Answer from the drawing. Dimensions are ordinates in mm from the lowest x, y and z of the part. A direction names the side the tool comes from. Round coordinates to 2 decimals unless told otherwise and drop trailing zeros. Loops run counter-clockwise (first coordinate to the right, second up) from the corner with the lowest first, then second, coordinate; pieces in that order, holes last.
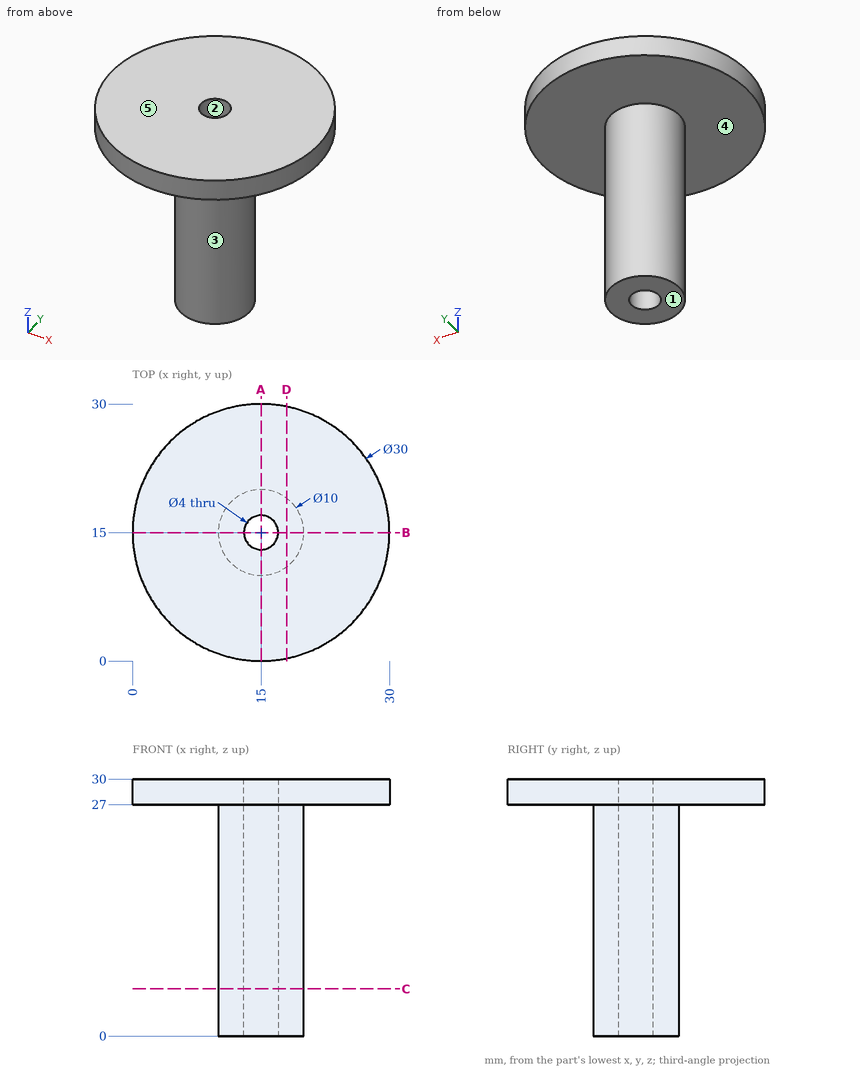
Item 1: For the marked faces 4 and 5, determine the directions among +Z, -Z, +X, -X, +Y, -Y from which every point of the face is accessible in a straight line to the end or side of a thin tool.
Item 2: Straight lines are drawn through the part: line 1 (Z direction, x = 12.5, y = 2.25); line 2 (Y direction, x = 15, z = 16); line 3 (X direction, y = 15.5, z = 16.5). For each, find the intervals that lie inside material, in ascending order.
Item 3: Section A-A, the plane x = 15 is taken. Give the vertices of the cut face in (y, z).
Item 4: Section C-C, the plane z = 5.5 is taken. Give the vertices of the cut face in (x, y), plus the area to 3 significant figures.
Item 5: Determine the mould class of the marked faces 1, 2 and 3 for opening direction Y: pulls with the +Y half, pulls with the -Y half, needs draft (parallel to the pull), parting line crosses it, or undercut.
Item 6: Section D-D, the plane x = 18 is taken. Give the vertices of the cut face in (y, z), plus the area to 3 significant figures.
Item 7: This flat-tipped pin is pushed along its axis until it touches: P1, Ø2, axis at x = 16.5, z = 7.5, coming from the -Y side. Where does it stop, or does it pass through?
Answer below:
1. face 4: -Z
1. face 5: +Z, +X, -X, +Y, -Y
2. line 1: z = 27 to 30
2. line 2: y = 10 to 13, 17 to 20
2. line 3: x = 10.03 to 13.06, 16.94 to 19.97
3. outline: (0, 27) - (10, 27) - (10, 0) - (13, 0) - (13, 30) - (0, 30) - close; (17, 0) - (20, 0) - (20, 27) - (30, 27) - (30, 30) - (17, 30) - close
4. outline: circle Ø10 at (15, 15); hole circle Ø4 at (15, 15)
4. area: 66.0 mm2
5. face 1: needs draft
5. face 2: undercut
5. face 3: parting line crosses it
6. outline: (0.3, 27) - (11, 27) - (11, 0) - (19, 0) - (19, 27) - (29.7, 27) - (29.7, 30) - (0.3, 30) - close
6. area: 304 mm2
7. P1: stops at y = 10.03
